```python
from build123d import *

# Parameters (mm, degrees)
BOSS_EXTRU_1_DEPTH      = 6
ENL_V_MAT_EXTRU_1_DEPTH = 10


with BuildPart() as part:
    # Esquisse1 → Boss.-Extru.1 (new body)
    with BuildSketch(Plane.XY):
        Polygon((-40.636697438, 45.053641116), (-40.636697438, 39.053641116), (-42.636697438, 39.053641116), (-42.636697438, -160.946358884), (-40.636697438, -160.946358884), (-40.636697438, -166.946358884), (-34.636697438, -166.946358884), (-34.636697438, -160.946358884), (-32.636697438, -160.946358884), (-32.636697438, -157.946358884), (-34.136697438, -157.946358884), (-34.136697438, -154.946358884), (-32.636697438, -154.946358884), (-32.636697438, -150.946358884), (-28.636697438, -150.946358884), (-28.636697438, -154.946358884), (-27.136697438, -154.946358884), (-27.136697438, -157.946358884), (-28.636697438, -157.946358884), (-28.636697438, -160.946358884), (-26.636697438, -160.946358884), (-26.636697438, -166.946358884), (-20.636697438, -166.946358884), (-20.636697438, -160.946358884), (3.863302562, -160.946358884), (3.863302562, -60.946358884), (6.863302562, -60.946358884), (6.863302562, 39.053641116), (-20.636697438, 39.053641116), (-20.636697438, 45.053641116), (-26.636697438, 45.053641116), (-26.636697438, 39.053641116), (-28.636697438, 39.053641116), (-28.636697438, 36.053641116), (-27.136697438, 36.053641116), (-27.136697438, 33.053641116), (-28.636697438, 33.053641116), (-28.636697438, 29.053641116), (-32.636697438, 29.053641116), (-32.636697438, 33.053641116), (-34.136697438, 33.053641116), (-34.136697438, 36.053641116), (-32.636697438, 36.053641116), (-32.636697438, 39.053641116), (-34.636697438, 39.053641116), (-34.636697438, 45.053641116), align=None)
        Polygon((34.363302562, 39.053641116), (6.863302562, 39.053641116), (6.863302562, -60.946358884), (9.863302562, -60.946358884), (9.863302562, -160.946358884), (34.363302562, -160.946358884), (34.363302562, -166.946358884), (40.363302562, -166.946358884), (40.363302562, -160.946358884), (42.363302562, -160.946358884), (42.363302562, -157.946358884), (40.863302562, -157.946358884), (40.863302562, -154.946358884), (42.363302562, -154.946358884), (42.363302562, -150.946358884), (46.363302562, -150.946358884), (46.363302562, -154.946358884), (47.863302562, -154.946358884), (47.863302562, -157.946358884), (46.363302562, -157.946358884), (46.363302562, -160.946358884), (48.363302562, -160.946358884), (48.363302562, -166.946358884), (54.363302562, -166.946358884), (54.363302562, -160.946358884), (56.363302562, -160.946358884), (56.363302562, 39.053641116), (54.363302562, 39.053641116), (54.363302562, 45.053641116), (48.363302562, 45.053641116), (48.363302562, 39.053641116), (46.363302562, 39.053641116), (46.363302562, 36.053641116), (47.863302562, 36.053641116), (47.863302562, 33.053641116), (46.363302562, 33.053641116), (46.363302562, 29.053641116), (42.363302562, 29.053641116), (42.363302562, 33.053641116), (40.863302562, 33.053641116), (40.863302562, 36.053641116), (42.363302562, 36.053641116), (42.363302562, 39.053641116), (40.363302562, 39.053641116), (40.363302562, 45.053641116), (34.363302562, 45.053641116), align=None)
    extrude(amount=BOSS_EXTRU_1_DEPTH)

    # Esquisse2 → Enlèv. mat.-Extru.1 (cut)
    with BuildSketch(Plane.XY.offset(6)):
        with BuildLine():
            Line((-20.636697438, 39.053641116), (34.363302562, 39.053641116))
            ThreePointArc((34.363302562, 39.053641116), (6.863302562, 17.053641116), (-20.636697438, 39.053641116))
        make_face()
    extrude(amount=-ENL_V_MAT_EXTRU_1_DEPTH, mode=Mode.SUBTRACT)


solid = part.part
```
For this review, take the finished solid that the model builds, in its own axes (mm). A direction names the side the tool comes from. Give positions to 0.01 mm unless a question says otherwise; leave off trailing zeros. Write each loop counter-clockwise with the first axis right and the second up, starting at its lowest first coordinate (ties: lowest second). Pieces come first, ordered by that corner, then holes. Notation, with made-up numbers: M -23.75,20 L -18.75,20 A24 cw -18.75,40 Z; hole C 64.25,86 d4. An arc over 180 degrees is marked long. One line per item, written item: value.
1) Take a section at C-C, the plane x = -15.5. Write out the cut boundary in (y, z).
Results are:
outline: M -160.95,0 L 28.08,0 L 28.08,6 L -160.95,6 Z
2) For P1, Ø3, axis at x = 45, z = 3.5, coming from the +Y side; P2, Ø1.2, axis at x = 44.5, z = 3.5, coming from the -Y side; P3, Ø2, axis at x = 27, y = -34.5, coming from the -Z side; P4, Ø1.8, axis at y = 41, z = 3.5, coming from the -X side, all flat-tipped, find the tip position at first contact; note any pin that passes through.
Results are:
P1: stops at y = 39.05
P2: stops at y = -150.95
P3: stops at z = 0
P4: stops at x = -40.64
3) The part is to be moulded in two halves that separate along X. For faces 1 (the flat face through (46.363, -153, 3)), 2 (the flat face through (44, 29.054, 3)), 3 (the flat face through (-24, -166.946, 3)), 4 (the flat face through (-40.637, 42, 3)), say which applies: +X half, -X half, draft (parallel to the pull), parting line (faces both ways), or undercut.
Results are:
face 1: undercut
face 2: undercut
face 3: draft
face 4: -X half
4) Take a section at A-A, the plane y = -110. Write out the cut boundary in (x, z), then the cut area to 3 significant figures.
Results are:
outline: M -42.64,0 L 3.86,0 L 3.86,6 L -42.64,6 Z; M 9.86,0 L 56.36,0 L 56.36,6 L 9.86,6 Z
area: 558 mm²
5) For line 1 (X direction, y = -152, z = 2.4); line 2 (X direction, y = -156, z = 2.3); line 3 (Y direction, x = -28.5, z = 3.4), list the stretches that pass through material, from the lowest coordinate up. Write a range as from..to.
Results are:
line 1: x = -42.64..-32.64, -28.64..3.86, 9.86..42.36, 46.36..56.36
line 2: x = -42.64..-34.14, -27.14..3.86, 9.86..40.86, 47.86..56.36
line 3: y = -160.95..-157.95, -154.95..33.05, 36.05..39.05
6) Take a section at B-B, the plane y = 25. Write out the cut boundary in (x, z), then the cut area to 3 significant figures.
Results are:
outline: M -42.64,0 L -12.75,0 L -12.75,6 L -42.64,6 Z; M 26.48,0 L 56.36,0 L 56.36,6 L 26.48,6 Z
area: 359 mm²
7) For faces 5 (the flat face through (-26.637, 42, 3)), 6 (the flat face through (9.863, -110, 3)), 7 (the flat face through (6, -59, 6)), list the 3-axis set-ups (+Z, -Z, +X, -X, +Y, -Y) from which the entire face can be reached by the end or side of a thin tool; tool diameter is ignored.
Results are:
face 5: +Z, -Z, +Y
face 6: +Z, -Z, -Y
face 7: +Z, +X, -X, +Y, -Y
